```python
from build123d import *

# Parameters (mm, degrees)
SKETCH1_W           = 182
SKETCH1_H           = 62
BOSS_EXTRUDE1_DEPTH = 5
SKETCH2_W           = 145
SKETCH2_H           = 5
BOSS_EXTRUDE2_DEPTH = 18
SKETCH3_R           = 2
CUT_EXTRUDE1_DEPTH  = 18
SKETCH4_W           = 7
SKETCH4_H           = 62
BOSS_EXTRUDE3_DEPTH = 78
SKETCH5_W           = 175
SKETCH5_H           = 7
BOSS_EXTRUDE4_DEPTH = 78
SKETCH6_W           = 7
SKETCH6_H           = 19
BOSS_EXTRUDE5_DEPTH = 18.5
SKETCH7_R           = 2
CUT_EXTRUDE2_DEPTH  = 18
SKETCH8_W           = 7
SKETCH8_H           = 8.2
CUT_EXTRUDE3_DEPTH  = 2.3
SKETCH11_R          = 1.5
SKETCH11_W          = 34
SKETCH11_H          = 26
CUT_EXTRUDE5_DEPTH  = 10
SKETCH12_W          = 5
SKETCH12_H          = 55
BOSS_EXTRUDE6_DEPTH = 10
SKETCH13_W          = 5
SKETCH13_H          = 10
BOSS_EXTRUDE7_DEPTH = 63
SKETCH15_R          = 2
CUT_EXTRUDE6_DEPTH  = 63
SKETCH16_R          = 3
CUT_EXTRUDE7_DEPTH  = 10
SKETCH17_R          = 2
CUT_EXTRUDE8_DEPTH  = 10
SKETCH18_R          = 1.5
CUT_EXTRUDE9_DEPTH  = 10


with BuildPart() as part:
    # Sketch1 → Boss-Extrude1 (new body)
    with BuildSketch(Plane(origin=(0, 0, 0), x_dir=(1, 0, 0), z_dir=(0, 1, 0))):
        with Locations((46.151515152, -7.666666667)):
            Rectangle(SKETCH1_W, SKETCH1_H)
    extrude(amount=BOSS_EXTRUDE1_DEPTH)

    # Sketch2 → Boss-Extrude2 (add)
    with BuildSketch(Plane(origin=(0, 5, 0), x_dir=(1, 0, 0), z_dir=(0, 1, 0))):
        with Locations((49.651515152, -36.166666667)):
            Rectangle(SKETCH2_W, SKETCH2_H)
    extrude(amount=BOSS_EXTRUDE2_DEPTH)

    # Sketch3 → Cut-Extrude1 (cut)
    with BuildSketch(Plane(origin=(0, 0, 33.666666667), x_dir=(-1, 0, 0), z_dir=(0, 0, -1))):
        with Locations((-102.151515152, 14.1)):
            Circle(SKETCH3_R)
        with Locations((-49.651515152, 14.1)):
            Circle(SKETCH3_R)
        with Locations((2.848484848, 14.1)):
            Circle(SKETCH3_R)
    extrude(amount=-CUT_EXTRUDE1_DEPTH, mode=Mode.SUBTRACT)

    # Sketch4 → Boss-Extrude3 (add)
    with BuildSketch(Plane(origin=(0, 5, 0), x_dir=(1, 0, 0), z_dir=(0, 1, 0))):
        with Locations((-41.348484848, -7.666666667)):
            Rectangle(SKETCH4_W, SKETCH4_H)
    extrude(amount=BOSS_EXTRUDE3_DEPTH)

    # Sketch5 → Boss-Extrude4 (add)
    with BuildSketch(Plane(origin=(0, 5, 0), x_dir=(1, 0, 0), z_dir=(0, 1, 0))):
        with Locations((49.651515152, 19.833333333)):
            Rectangle(SKETCH5_W, SKETCH5_H)
    extrude(amount=BOSS_EXTRUDE4_DEPTH)

    # Sketch6 → Boss-Extrude5 (add)
    with BuildSketch(Plane.XY.offset(38.666666667)):
        with Locations((-41.348484848, 52.5)):
            Rectangle(SKETCH6_W, SKETCH6_H)
    extrude(amount=BOSS_EXTRUDE5_DEPTH)

    # Sketch7 → Cut-Extrude2 (cut)
    with BuildSketch(Plane(origin=(0, 62, 0), x_dir=(1, 0, 0), z_dir=(0, 1, 0))):
        with Locations((-41.348484848, -48.666666667)):
            Circle(SKETCH7_R)
    extrude(amount=-CUT_EXTRUDE2_DEPTH, mode=Mode.SUBTRACT)

    # Sketch8 → Cut-Extrude3 (cut)
    with BuildSketch(Plane.XZ.offset(-43)):
        with Locations((-41.348484848, 48.666666667)):
            Rectangle(SKETCH8_W, SKETCH8_H)
    extrude(amount=-CUT_EXTRUDE3_DEPTH, mode=Mode.SUBTRACT)

    # Sketch11 → Cut-Extrude5 (cut)
    with BuildSketch(Plane(origin=(-37.848484848, 0, 0), x_dir=(0, 0, -1), z_dir=(1, 0, 0))):
        with Locations((-20.666666667, 74.5)):
            Circle(SKETCH11_R)
        with Locations((-0.666666667, 70)):
            Rectangle(SKETCH11_W, SKETCH11_H)
    extrude(amount=-CUT_EXTRUDE5_DEPTH, mode=Mode.SUBTRACT)

    # Sketch12 → Boss-Extrude6 (add)
    with BuildSketch(Plane(origin=(0, 5, 0), x_dir=(1, 0, 0), z_dir=(0, 1, 0))):
        with Locations((134.651515152, -11.166666667)):
            Rectangle(SKETCH12_W, SKETCH12_H)
    extrude(amount=BOSS_EXTRUDE6_DEPTH)

    # Sketch13 → Boss-Extrude7 (add)
    with BuildSketch(Plane(origin=(0, 15, 0), x_dir=(1, 0, 0), z_dir=(0, 1, 0))):
        with Locations((134.651515152, 11.333333333)):
            Rectangle(SKETCH13_W, SKETCH13_H)
    extrude(amount=BOSS_EXTRUDE7_DEPTH)

    # Sketch15 → Cut-Extrude6 (cut)
    with BuildSketch(Plane(origin=(137.151515152, 0, 0), x_dir=(0, 0, -1), z_dir=(1, 0, 0))):
        with Locations((11.333333333, 65)):
            Circle(SKETCH15_R)
        with Locations((11.333333333, 40)):
            Circle(SKETCH15_R)
        with Locations((11.333333333, 10)):
            Circle(SKETCH15_R)
        with Locations((-28.666666667, 10)):
            Circle(SKETCH15_R)
        with Locations((-9.666666667, 10)):
            Circle(SKETCH15_R)
    extrude(amount=-CUT_EXTRUDE6_DEPTH, mode=Mode.SUBTRACT)

    # Sketch16 → Cut-Extrude7 (cut)
    with BuildSketch(Plane(origin=(0, 0, -23.333333333), x_dir=(-1, 0, 0), z_dir=(0, 0, -1))):
        with Locations((-77.151515152, 40)):
            Circle(SKETCH16_R)
        with Locations((-77.151515152, 63)):
            Circle(SKETCH16_R)
    extrude(amount=-CUT_EXTRUDE7_DEPTH, mode=Mode.SUBTRACT)

    # Sketch17 → Cut-Extrude8 (cut)
    with BuildSketch(Plane(origin=(0, 0, -23.333333333), x_dir=(-1, 0, 0), z_dir=(0, 0, -1))):
        with Locations((20.848484848, 68)):
            Circle(SKETCH17_R)
        with Locations((20.848484848, 38)):
            Circle(SKETCH17_R)
        with Locations((-4.151515152, 38)):
            Circle(SKETCH17_R)
        with Locations((-4.151515152, 68)):
            Circle(SKETCH17_R)
    extrude(amount=-CUT_EXTRUDE8_DEPTH, mode=Mode.SUBTRACT)

    # Sketch18 → Cut-Extrude9 (cut)
    with BuildSketch(Plane(origin=(-37.848484848, 0, 0), x_dir=(0, 0, -1), z_dir=(1, 0, 0))):
        with Locations((12.333333333, 10)):
            Circle(SKETCH18_R)
        with Locations((-21.666666667, 10)):
            Circle(SKETCH18_R)
    extrude(amount=-CUT_EXTRUDE9_DEPTH, mode=Mode.SUBTRACT)


solid = part.part
```
Source: CAD feature listing. Evaluate the final solid. Frame: model axes, mm. A direction names the side the tool comes from. Round coordinates to 2 decimals unless told otherwise and drop trailing zeros. Loops run counter-clockwise (first coordinate to the right, second up) from the corner with the lowest first, then second, coordinate; pieces in that order, holes last. Notation, with made-up numbers: M 86,22 L 94,22 A32 ccw 94,55 Z; hole C 15.5,-15.75 d4. An arc over 180 degrees is marked long. Put each result on its own line as item: value.
(1) First-contact query: pin 1 (12 mm diameter, centred on x = 70, z = -2.5, fed in from +Y); pin 2 (3.5 mm diameter, centred on x = -40.5, z = 54.5, fed in from -Y); pin 3 (4 mm diameter, centred on x = 113, y = 70.5, fed in from +Z). Flat tips, straight axial feed; report the tip coordinate or a pass-through.
Solutions:
pin 1: y = 5
pin 2: y = 43
pin 3: z = -16.33
(2) Ray query, line 1 (X direction, y = 14, z = 31.5); line 2 (Z direction, x = -20, y = 10.5); line 3 (Y direction, x = 7, z = -2). Return the intervals inside material, ascending. Write a range as [from, to].
Solutions:
line 1: [-44.85, -37.85], [132.15, 137.15]
line 2: [-23.33, -16.33], [33.67, 38.67]
line 3: [0, 5]
(3) Access query for faces 4 (the face through (135, 78, -11)), 5 (the face through (49, 23, 36)), 6 (the face through (-41, 70, 17.667)), 7 (the face through (134.687, 10.088, 30.665)), 8 (the face through (132.152, 31, -7)). Directions: +Z, -Z, +X, -X, +Y, -Y. A direction counts if a zero-diameter tool reaches every point of the face in a straight line with its end or side. Return the directions, or none.
Solutions:
face 4: +Z, +X, -X, +Y
face 5: +Z, +X, +Y
face 6: +X, -X, +Y
face 7: +X
face 8: +Z, +Y
(4) Section D-D, the plane x = 76. Return loops of the section in (y, z).
Solutions:
outline: M 0,-23.33 L 37.23,-23.33 L 37.23,-16.33 L 5,-16.33 L 5,33.67 L 23,33.67 L 23,38.67 L 0,38.67 Z; M 42.77,-23.33 L 60.23,-23.33 L 60.23,-16.33 L 42.77,-16.33 Z; M 65.77,-23.33 L 83,-23.33 L 83,-16.33 L 65.77,-16.33 Z
(5) Pull-direction query (Y, two-part tool) for faces 1 (the face through (45, 0, 7)), 2 (the face through (134.687, 11.983, -11.073)), 3 (the face through (122.152, 14, 36)); classes: released by +Y, released by -Y, zero draft, split by the parting line, or undercut.
Solutions:
face 1: released by -Y
face 2: undercut
face 3: zero draft
(6) Section C-C, the plane y = 47.5. Return loops of the section in (x, z), and give its area (3 significant figures).
Solutions:
outline: M -44.85,-23.33 L 137.15,-23.33 L 137.15,-6.33 L 132.15,-6.33 L 132.15,-16.33 L -37.85,-16.33 L -37.85,57.17 L -44.85,57.17 Z; hole C -41.35,48.67 d4
area: 1,830 mm²
(7) Section A-A, the plane y = 18. Return loops of the section in (x, z).
Solutions:
outline: M -44.85,-23.33 L 137.15,-23.33 L 137.15,-6.33 L 132.15,-6.33 L 132.15,-16.33 L -37.85,-16.33 L -37.85,38.67 L -44.85,38.67 Z; M -22.85,33.67 L 122.15,33.67 L 122.15,38.67 L -22.85,38.67 Z
(8) Section B-B, the plane x = 38. Return loops of the section in (y, z), and give its area (3 significant figures).
Solutions:
outline: M 0,-23.33 L 83,-23.33 L 83,-16.33 L 5,-16.33 L 5,33.67 L 23,33.67 L 23,38.67 L 0,38.67 Z
area: 946 mm²
